Can you work these out from the model? Positions are in its coordinate system, mm. Face numbers are marked on the shaded views. A direction names the side the tool comes from. Round coordinates to 2 decimals unless told otherwise and drop trailing zeros. Write each loop counter-clockwise with the first axis right and the second up, starting at its lowest first coordinate (ties: lowest second). Pieces come first, ordered by that corner, then holes. Notation, with made-up numbers: M 28,54 L 59,54 A31 ccw 59,90 Z; hole C 46,42.25 d10. An arc over 180 degrees is marked long. Answer as a JSON object with one key per item and string values. Group by question number.
1) Please list where these lines run through material, in increasing order: L1, parallel to Z at x = -6, y = -5; L2, parallel to Y at x = 3, z = 3; L3, parallel to X at y = 6, z = 6. Write a range as [from, to].
2) Suppose I cut it at C-C, the plane y = 25. Write out the boundary of the cut face in (x, z), and give its area (3 significant figures).
3) I'm going to push flat-ended pins straight in: pin 1 Ø8 at (x, y) = (2, 37) entering from -Z; pin 2 Ø1 at (x, z) = (-8.5, 3.5) entering from +Y; pin 3 Ø5 at (x, y) = (2.5, 26.5) entering from -Z. Where does each tip first touch, or does it pass through?
4) If we mould it in two halves opening along Y, with no side actions, what happens to the marked faces 4, 5 and 6? For each: +Y half, -Y half, draft (parallel to the pull), parting line (faces both ways), or undercut.
5) Suppose I cut it at A-A, the plane x = -9.5. Write out the boundary of the cut face in (y, z), and give its area (3 significant figures).
6) Suppose I cut it at B-B, the plane y = 18. Write out the boundary of the cut face in (x, z) (3 decimals).
7) On a 3-axis mill with a long thin cutter (end or side, diameter ignored), from which of +Z, -Z, +X, -X, +Y, -Y can I reach the whole of each face in a straight line? I mean the marked faces 1, 2 and 3. Say none if no direction works.
8) Suppose I cut it at D-D, the plane x = 10. Write out the boundary of the cut face in (y, z).
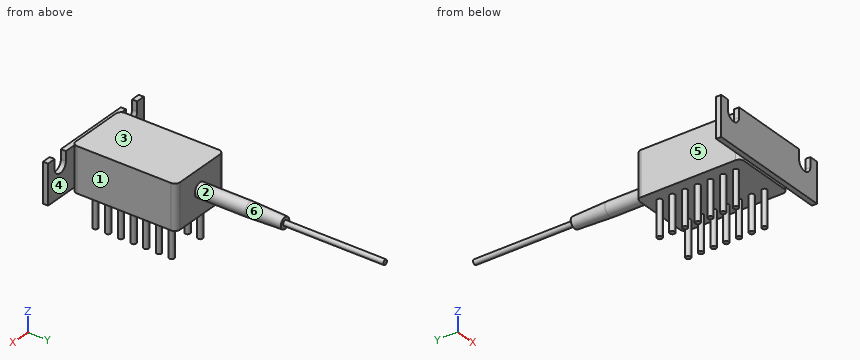
from build123d import *

# Parameters (mm, degrees)
SKETCH_1_W          = 12.7
SKETCH_1_H          = 20.8
EXTRUDE_1_DEPTH     = 8.9
SKETCH_2_R          = 0.5
EXTRUDE_2_DEPTH     = 7
FILLET_1_R          = 1
SKETCH_3_W          = 25.54
SKETCH_3_H          = 7.9
EXTRUDE_3_DEPTH     = 1
CUT_EXTRUDE_1_DEPTH = 27.786617928
SKETCH_5_R          = 1.375
EXTRUDE_4_DEPTH     = 17
CHAMFER_1_SIZE      = 7
CHAMFER_1_SIZE2     = 0.244445386
SKETCH_7_R          = 0.5
EXTRUDE_5_DEPTH     = 20


with BuildPart() as part:
    # 草图1 → 凸台-拉伸1 (new body)
    with BuildSketch(Plane.XY):
        Rectangle(SKETCH_1_W, SKETCH_1_H)
    extrude(amount=EXTRUDE_1_DEPTH)

    # 草图2 → 凸台-拉伸2 (add)
    with BuildSketch(Plane(origin=(0, 0, 0), x_dir=(-1, 0, 0), z_dir=(0, 0, -1))):
        with Locations(Location((-3.81, 0, 0), (0, 0, 180))):
            Circle(SKETCH_2_R)
        with Locations(Location((-3.81, 2.54, 0), (0, 0, 180))):
            Circle(SKETCH_2_R)
        with Locations(Location((-3.81, 5.08, 0), (0, 0, 180))):
            Circle(SKETCH_2_R)
        with Locations(Location((-3.81, 7.62, 0), (0, 0, 180))):
            Circle(SKETCH_2_R)
        with Locations(Location((-3.81, -2.54, 0), (0, 0, 180))):
            Circle(SKETCH_2_R)
        with Locations(Location((-3.81, -5.08, 0), (0, 0, 180))):
            Circle(SKETCH_2_R)
        with Locations(Location((-3.81, -7.62, 0), (0, 0, 180))):
            Circle(SKETCH_2_R)
        with Locations(Location((3.81, -7.62, 0), (0, 0, 180))):
            Circle(SKETCH_2_R)
        with Locations(Location((3.81, -5.08, 0), (0, 0, 180))):
            Circle(SKETCH_2_R)
        with Locations(Location((3.81, -2.54, 0), (0, 0, 180))):
            Circle(SKETCH_2_R)
        with Locations(Location((3.81, 7.62, 0), (0, 0, 180))):
            Circle(SKETCH_2_R)
        with Locations(Location((3.81, 5.08, 0), (0, 0, 180))):
            Circle(SKETCH_2_R)
        with Locations(Location((3.81, 2.54, 0), (0, 0, 180))):
            Circle(SKETCH_2_R)
        with Locations(Location((3.81, 0, 0), (0, 0, 180))):
            Circle(SKETCH_2_R)
    extrude(amount=EXTRUDE_2_DEPTH)

    # 圆角1
    fillet_1_edges = [part.edges().sort_by_distance(p)[0] for p in [
        (-6.35, 10.4, 4.45),
        (6.35, 10.4, 4.45),
        (6.35, -10.4, 4.45),
        (-6.35, -10.4, 4.45),
    ]]
    fillet(fillet_1_edges, radius=FILLET_1_R)

    # 草图3 → 凸台-拉伸3 (add)
    with BuildSketch(Plane.XZ.offset(10.4)):
        with Locations((0, 4.45)):
            Rectangle(SKETCH_3_W, SKETCH_3_H)
    extrude(amount=EXTRUDE_3_DEPTH)

    # 草图4 → 切除-拉伸1 (cut, through all)
    with BuildSketch(Plane.XZ.offset(11.4)):
        with BuildLine():
            Line((8, 6.5), (8, 8.4))
            Line((8, 8.4), (11, 8.4))
            Line((11, 8.4), (11, 6.5))
            ThreePointArc((11, 6.5), (9.5, 5), (8, 6.5))
        make_face()
        with BuildLine():
            Line((-8, 8.4), (-11, 8.4))
            Line((-11, 8.4), (-11, 6.5))
            ThreePointArc((-11, 6.5), (-9.5, 5), (-8, 6.5))
            Line((-8, 6.5), (-8, 8.4))
        make_face()
    extrude(amount=-CUT_EXTRUDE_1_DEPTH, mode=Mode.SUBTRACT)

    # 草图5 → 凸台-拉伸4 (add)
    with BuildSketch(Plane(origin=(0, 10.4, 0), x_dir=(1, 0, 0), z_dir=(0, 1, 0))):
        with Locations(Location((0, -4.9, 0), (0, 0, 90))):
            Circle(SKETCH_5_R)
    extrude(amount=EXTRUDE_4_DEPTH)

    # 倒角1
    chamfer_1_edges = [part.edges().sort_by_distance(p)[0] for p in [
        (0, 27.4, 6.275),
    ]]
    chamfer_1_side = [part.faces().sort_by_distance(p)[0] for p in [
        (0, 18.9, 6.275),
    ]]
    chamfer(chamfer_1_edges, length=CHAMFER_1_SIZE, length2=CHAMFER_1_SIZE2, reference=chamfer_1_side[0])

    # 草图7 → 凸台-拉伸5 (add)
    with BuildSketch(Plane(origin=(0, 27.4, 0), x_dir=(1, 0, 0), z_dir=(0, 1, 0))):
        with Locations(Location((0, -4.9, 0), (0, 0, 270))):
            Circle(SKETCH_7_R)
    extrude(amount=EXTRUDE_5_DEPTH)


solid = part.part
Results:
{
 "1": {"L1": "[0, 8.9]", "L2": "[-11.4, 10.4]", "L3": "[-6.35, 6.35]"},
 "2": {"outline": "C 0,4.9 d2.43", "area": "4.63 mm^2"},
 "3": {"pin 1": "z = 4.4", "pin 2": "y = -10.4", "pin 3": "z = 3.72"},
 "4": {"face 4": "undercut", "face 5": "draft", "face 6": "+Y half"},
 "5": {"outline": "M -11.4,0.5 L -10.4,0.5 L -10.4,5 L -11.4,5 Z", "area": "4.50 mm^2"},
 "6": {"outline": "C 0,4.9 d2.75"},
 "7": {"face 1": "+Z, -Z, +X, +Y", "face 2": "+Y", "face 3": "+Z, +X, -X, +Y, -Y"},
 "8": {"outline": "M -11.4,0.5 L -10.4,0.5 L -10.4,5.09 L -11.4,5.09 Z"}
}
